```python
from build123d import *

# Parameters (mm, degrees)
SKETCH1_W           = 368.3
SKETCH1_H           = 165.1
BOSS_EXTRUDE1_DEPTH = 6.35
SKETCH2_R           = 52.705
SKETCH2_R_2         = 2.0828
SKETCH2_W           = 129.54
SKETCH2_H           = 32.004
CUT_EXTRUDE1_DEPTH  = 202.906036314


with BuildPart() as part:
    # Sketch1 → Boss-Extrude1 (new body)
    with BuildSketch(Plane(origin=(0, 0, 0), x_dir=(1, 0, 0), z_dir=(0, 1, 0))):
        Rectangle(SKETCH1_W, SKETCH1_H)
    extrude(amount=BOSS_EXTRUDE1_DEPTH)

    # Sketch2 → Cut-Extrude1 (cut, through all)
    with BuildSketch(Plane(origin=(0, 6.35, 0), x_dir=(1, 0, 0), z_dir=(0, 1, 0))):
        with Locations(Location((92.075, 0, 0), (0, 0, 270))):
            Circle(SKETCH2_R)
        with Locations(Location((-159.0294, 18.1864, 0), (0, 0, 270))):
            Circle(SKETCH2_R_2)
        with Locations(Location((-159.0294, -18.1864, 0), (0, 0, 90))):
            Circle(SKETCH2_R_2)
        with Locations(Location((-25.1206, 18.1864, 0), (0, 0, 90))):
            Circle(SKETCH2_R_2)
        with Locations(Location((-25.1206, -18.1864, 0), (0, 0, 270))):
            Circle(SKETCH2_R_2)
        with Locations((-92.075, 0)):
            Rectangle(SKETCH2_W, SKETCH2_H)
    extrude(amount=-CUT_EXTRUDE1_DEPTH, mode=Mode.SUBTRACT)


solid = part.part
```
Part model, mm, in its own coordinate system. A direction names the side the tool comes from. Round coordinates to 2 decimals unless told otherwise and drop trailing zeros. Write each loop counter-clockwise with the first axis right and the second up, starting at its lowest first coordinate (ties: lowest second). Pieces come first, ordered by that corner, then holes. Notation, with made-up numbers: (-38.5, 28) -> (-8.5, 28) arc R6 cw to (-8.5, 38) -> close; hole circle Ø4 at (44.5, 0). An arc over 180 degrees is marked (long way). Return JSON: item names as keys, results as strings. Group by question number.
Q1. Probe L1, parallel to X at y = 4, z = 1 (3 decimals); L2, parallel to X at y = 5.5, z = -14.5 (3 decimals); L3, parallel to Z at x = 83.5, y = 2. List the from-to ranges inside material, lowest first. Write a range as [from, to].
Q2. Saw through at C-C on z = -24. Write the cut outline in (x, y).
Q3. Saw through at B-B on x = -100.5. Write the cut outline in (y, z), plus the area to 3 significant figures.
Q4. Saw through at A-A on z = 0. Write the cut outline in (x, y) (3 decimals).
Q5. Saw through at D-D on y = 1.5. Write the cut outline in (x, z) (3 decimals).
Q6. Pin check, flat tip, straight feed: pin 1 (3.5 mm diameter, centred on x = -159.03, z = -18.19, fed in from +Y). Stop position of the tip, or through.
Q7. Which spindle directions (+Z, -Z, +X, -X, +Y, -Y) get a long thin tool onto all of the face, cutting with end or side? Do faces 1 (the flat face through (-93, 3, 16.002)), 2 (the flat face through (-184.15, 3, 1)). Say none if no direction does.
Q8. Mould opens along Z. For faces 3 (the flat face through (-3, 6.35, -1)), 4 (the flat face through (-3, 3, -82.55)), 5 (the flat face through (-93, 3, -16.002)) say: pulls with the +Z half, pulls with the -Z half, needs draft (parallel to the pull), parting line crosses it, or undercut.
Answer:
{
 "1": {"L1": "[-184.15, -156.845], [-27.305, 39.379], [144.771, 184.15]", "L2": "[-184.15, -156.845], [-27.305, 41.404], [142.746, 184.15]", "L3": "[-82.55, -52], [52, 82.55]"},
 "2": {"outline": "(-184.15, 0) -> (45.15, 0) -> (45.15, 6.35) -> (-184.15, 6.35) -> close; (139, 0) -> (184.15, 0) -> (184.15, 6.35) -> (139, 6.35) -> close"},
 "3": {"outline": "(0, -82.55) -> (6.35, -82.55) -> (6.35, -16) -> (0, -16) -> close; (0, 16) -> (6.35, 16) -> (6.35, 82.55) -> (0, 82.55) -> close", "area": "845 mm2"},
 "4": {"outline": "(-184.15, 0) -> (-156.845, 0) -> (-156.845, 6.35) -> (-184.15, 6.35) -> close; (-27.305, 0) -> (39.37, 0) -> (39.37, 6.35) -> (-27.305, 6.35) -> close; (144.78, 0) -> (184.15, 0) -> (184.15, 6.35) -> (144.78, 6.35) -> close"},
 "5": {"outline": "(-184.15, -82.55) -> (184.15, -82.55) -> (184.15, 82.55) -> (-184.15, 82.55) -> close; hole circle Ø4.166 at (-159.029, -18.186); hole circle Ø4.166 at (-159.029, 18.186); hole (-156.845, -16.002) -> (-27.305, -16.002) -> (-27.305, 16.002) -> (-156.845, 16.002) -> close; hole circle Ø4.166 at (-25.121, -18.186); hole circle Ø4.166 at (-25.121, 18.186); hole circle Ø105.41 at (92.075, 0)"},
 "6": {"pin 1": "through"},
 "7": {"face 1": "+Y, -Y", "face 2": "+Z, -Z, -X, +Y, -Y"},
 "8": {"face 3": "needs draft", "face 4": "pulls with the -Z half", "face 5": "undercut"}
}
